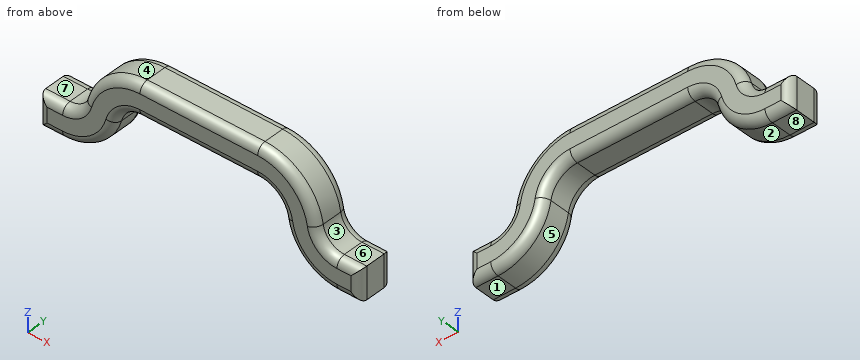
```python
from build123d import *

# Parameters (mm, degrees)
F1_DEPTH = 22.1615
F2_R     = 5.08


# Not quite as in the source:
# - a feature names something its author has since deleted; it is built from what else it names


with BuildPart() as f1:
    # F0 (on Front) → F1 (new body)
    with BuildSketch(Plane.XZ):
        with BuildLine():
            Line((28.6224108991, 72.15352447), (-41.2275891009, 72.15352447))
            ThreePointArc((-41.2275891009, 72.15352447), (-62.3757268242, 65.0226226894), (-74.8879136272, 46.5418578033))
            ThreePointArc((-74.8879136272, 46.5418578033), (-79.4377997374, 39.8215796629), (-87.1280316368, 37.22852447))
            Line((-87.1280316368, 37.22852447), (-101.5525891009, 37.22852447))
            Line((-101.5525891009, 37.22852447), (-101.5525891009, 18.17852447))
            Line((-101.5525891009, 18.17852447), (-87.1280316368, 18.17852447))
            ThreePointArc((-87.1280316368, 18.17852447), (-67.9024518883, 24.6611624523), (-56.5277366129, 41.4618578033))
            ThreePointArc((-56.5277366129, 41.4618578033), (-50.8403789751, 49.8622054788), (-41.2275891009, 53.10352447))
            Line((-41.2275891009, 53.10352447), (28.6224108991, 53.10352447))
            ThreePointArc((28.6224108991, 53.10352447), (38.9482036141, 49.2864525593), (44.3084160673, 39.6708321623))
            ThreePointArc((44.3084160673, 39.6708321623), (55.0288409738, 20.4395913682), (75.6804264037, 12.8054475469))
            Line((75.6804264037, 12.8054475469), (88.9474108991, 12.8054475469))
            Line((88.9474108991, 12.8054475469), (88.9474108991, 31.8554475469))
            Line((88.9474108991, 31.8554475469), (75.6804264037, 31.8554475469))
            ThreePointArc((75.6804264037, 31.8554475469), (67.4197922317, 34.9091050754), (63.1316222691, 42.601601393))
            ThreePointArc((63.1316222691, 42.601601393), (51.3391548721, 63.7559662665), (28.6224108991, 72.15352447))
        make_face()
    extrude(amount=F1_DEPTH)

    # F2
    f2_edges = [f1.edges().sort_by_distance(p)[0] for p in [
        (88.947411, -22.1615, 22.330448),
        (82.313919, -22.1615, 31.855448),
        (67.419792, -22.1615, 34.909105),
        (51.339155, -22.1615, 63.755966),
        (-6.302589, -22.1615, 72.153524),
        (-62.375727, -22.1615, 65.022623),
        (-79.4378, -22.1615, 39.82158),
        (-94.34031, -22.1615, 37.228524),
        (-101.552589, -22.1615, 27.703524),
        (-94.34031, -22.1615, 18.178524),
        (-67.902452, -22.1615, 24.661162),
        (-50.840379, -22.1615, 49.862205),
        (-6.302589, -22.1615, 53.103524),
        (38.948204, -22.1615, 49.286453),
        (55.028841, -22.1615, 20.439591),
        (82.313919, -22.1615, 12.805448),
        (88.947411, 0, 22.330448),
        (82.313919, 0, 31.855448),
        (67.419792, 0, 34.909105),
        (51.339155, 0, 63.755966),
        (-6.302589, 0, 72.153524),
        (-62.375727, 0, 65.022623),
        (-79.4378, 0, 39.82158),
        (-94.34031, 0, 37.228524),
        (-101.552589, 0, 27.703524),
        (-94.34031, 0, 18.178524),
        (-67.902452, 0, 24.661162),
        (-50.840379, 0, 49.862205),
        (-6.302589, 0, 53.103524),
        (38.948204, 0, 49.286453),
        (55.028841, 0, 20.439591),
        (82.313919, 0, 12.805448),
    ]]
    fillet(f2_edges, radius=F2_R)


solid = f1.part
```
Input: part model. Units: mm. Frame: model coordinates. Face numbers are marked on the shaded views. A direction names the side the tool comes from. Round coordinates to 2 decimals unless told otherwise and drop trailing zeros. Write each loop counter-clockwise with the first axis right and the second up, starting at its lowest first coordinate (ties: lowest second). Pieces come first, ordered by that corner, then holes. Notation, with made-up numbers: (62.25, 74) - (97.25, 74) arc R25 cw to (97.25, 89) - close; hole circle Ø8 at (36.25, 18.25). An arc over 180 degrees is marked (long way). Write item = value, one per line.
(1) Access query for the marked faces 5, 6, 7 and 8. Directions: +Z, -Z, +X, -X, +Y, -Y. A direction counts if a zero-diameter tool reaches every point of the face in a straight line with its end or side. Return the directions, or none.
Geometry check:
face_5 = -Z, +Y, -Y
face_6 = +Z, +X, +Y, -Y
face_7 = +Z, -X, +Y, -Y
face_8 = -Z, -X, +Y, -Y
(2) Contact query for flat-ended pins moving along their axis: pin 1 Ø9.5 at (x, y) = (80.5, -10) entering from +Z; pin 2 Ø1 at (y, z) = (-4.5, 56.5) entering from -X; pin 3 Ø8 at (x, z) = (54, 64.5) entering from +Y. Output: stop coordinate, or through.
Geometry check:
pin_1 = 31.86
pin_2 = -70.65
pin_3 = -1.31
(3) Section query C-C on y = -19.5. Output: boundary loops of the cut face in (x, z), then the cut area to 3 significant figures.
Geometry check:
outline = (-100.94, 18.79) - (-87.13, 18.79) arc R31.14 ccw to (-57.12, 41.63) arc R16.49 cw to (-41.23, 53.72) - (28.62, 53.72) arc R16.49 cw to (44.91, 39.77) arc R31.14 ccw to (75.68, 13.42) - (88.33, 13.42) - (88.33, 31.24) - (75.68, 31.24) arc R13.31 cw to (62.53, 42.51) arc R34.31 ccw to (28.62, 71.54) - (-41.23, 71.54) arc R34.31 ccw to (-74.3, 46.38) arc R13.31 cw to (-87.13, 36.62) - (-100.94, 36.62) - close
area = 4,020 mm^2
(4) Pull-direction query (X, two-part tool) for the marked faces 1, 2, 3 and 4; classes: +X half, -X half, draft (parallel to the pull), parting line (faces both ways), or undercut.
Geometry check:
face_1 = draft
face_2 = undercut
face_3 = +X half
face_4 = -X half
(5) Section query B-B on x = -29. Output: boundary loops of the cut face in (y, z), then the cut area to 3 significant figures.
Geometry check:
outline = (-22.16, 58.18) arc R5.08 ccw to (-17.08, 53.1) - (-5.08, 53.1) arc R5.08 ccw to (0, 58.18) - (0, 67.07) arc R5.08 ccw to (-5.08, 72.15) - (-17.08, 72.15) arc R5.08 ccw to (-22.16, 67.07) - close
area = 400 mm^2
(6) Section query A-A on y = -9.5. Output: boundary loops of the cut face in (x, z) (3 decimals), then the cut area to 3 significant figures.
Geometry check:
outline = (-101.553, 18.179) - (-87.128, 18.179) arc R31.75 ccw to (-56.528, 41.462) arc R15.875 cw to (-41.228, 53.104) - (28.622, 53.104) arc R15.875 cw to (44.308, 39.671) arc R31.75 ccw to (75.68, 12.805) - (88.947, 12.805) - (88.947, 31.855) - (75.68, 31.855) arc R12.7 cw to (63.132, 42.602) arc R34.925 ccw to (28.622, 72.154) - (-41.228, 72.154) arc R34.925 ccw to (-74.888, 46.542) arc R12.7 cw to (-87.128, 37.229) - (-101.553, 37.229) - close
area = 4,320 mm^2
(7) Material intervals for probe 1 along Z at (x, y) = (-42, -11.5); probe 2 along Z at (x, y) = (-39, -14); probe 3 along X at (y, z) = (-1.5, 51.5), sorted ascending.
Geometry check:
probe_1 = 53.08 to 72.14
probe_2 = 53.1 to 72.15
probe_3 = -71.48 to -51.1, 38.49 to 58.87
